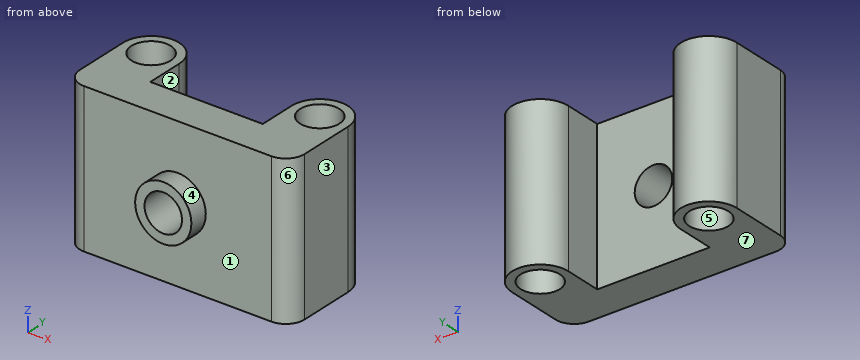
from build123d import *

# Parameters (mm, degrees)
SKETCH_1_W          = 12
SKETCH_1_H          = 8
EXTRUDE_1_DEPTH     = 2
EXTRUDE_6_DEPTH     = 8
SKETCH_11_R         = 1.05
CUT_EXTRUDE_1_DEPTH = 16.43534904
FILLET_3_R          = 1
SKETCH_12_R         = 1
CUT_EXTRUDE_2_DEPTH = 2
EXTRUDE_START       = 1
SKETCH_13_R         = 1.5
SKETCH_13_R_2       = 1
EXTRUDE_7_DEPTH     = 1


with BuildPart() as part:
    # 草图1 → 凸台-拉伸1 (new body)
    with BuildSketch(Plane(origin=(0, 0, 0), x_dir=(1, 0, 0), z_dir=(0, 1, 0))):
        with Locations((6, 0)):
            Rectangle(SKETCH_1_W, SKETCH_1_H)
    extrude(amount=EXTRUDE_1_DEPTH)

    # 草图10 → 凸台-拉伸6 (add)
    with BuildSketch(Plane(origin=(0, 0, -4), x_dir=(-1, 0, 0), z_dir=(0, 0, -1))):
        with BuildLine():
            Line((-12, 2), (-12, 4))
            ThreePointArc((-12, 4), (-10.5, 5.5), (-9, 4))
            Line((-9, 4), (-9, 2))
            Line((-9, 2), (-12, 2))
        make_face()
        with BuildLine():
            Line((-3, 2), (0, 2))
            Line((0, 2), (0, 4))
            ThreePointArc((0, 4), (-1.5, 5.5), (-3, 4))
            Line((-3, 4), (-3, 2))
        make_face()
    extrude(amount=-EXTRUDE_6_DEPTH)

    # 草图11 → 切除-拉伸1 (cut, through all)
    with BuildSketch(Plane(origin=(0, 0, -4), x_dir=(-1, 0, 0), z_dir=(0, 0, -1))):
        with Locations((-1.5, 4)):
            Circle(SKETCH_11_R)
        with Locations((-10.5, 4)):
            Circle(SKETCH_11_R)
    extrude(amount=-CUT_EXTRUDE_1_DEPTH, mode=Mode.SUBTRACT)

    # 圆角3
    fillet_3_edges = [part.edges().sort_by_distance(p)[0] for p in [
        (12, 0, 0),
        (0, 0, 0),
    ]]
    fillet(fillet_3_edges, radius=FILLET_3_R)

    # 草图12 → 切除-拉伸2 (cut)
    with BuildSketch(Plane.XZ):
        with Locations(Location((6, 0, 0), (0, 0, 270))):
            Circle(SKETCH_12_R)
    extrude(amount=-CUT_EXTRUDE_2_DEPTH, mode=Mode.SUBTRACT)

    # 草图13 → 凸台-拉伸7 (add)
    with BuildSketch(Plane.XZ.offset(EXTRUDE_START)):
        with Locations(Location((6, 0, 0), (0, 0, 90))):
            Circle(SKETCH_13_R)
        with Locations(Location((6, 0, 0), (0, 0, 270))):
            Circle(SKETCH_13_R_2, mode=Mode.SUBTRACT)
    extrude(amount=-EXTRUDE_7_DEPTH)


solid = part.part
For this review, take the finished solid that the model builds, in its own axes (mm). Face numbers are marked on the shaded views. A direction names the side the tool comes from. Round coordinates to 2 decimals unless told otherwise and drop trailing zeros. Loops run counter-clockwise (first coordinate to the right, second up) from the corner with the lowest first, then second, coordinate; pieces in that order, holes last. Notation, with made-up numbers: (-21, 78) - (-1, 78) arc R25 cw to (-1, 101) - close; hole circle Ø10 at (23, -25). An arc over 180 degrees is marked (long way). Put each result on its own line as item: value. Start each with the question number.
1. For the marked faces 1, 2 and 3, list the 3-axis set-ups (+Z, -Z, +X, -X, +Y, -Y) from which the entire face can be reached by the end or side of a thin tool; tool diameter is ignored.
2. Consider section D-D on z = -2.75. State the section outline as (x, y) points, plus the area to 3 significant figures.
3. Consider section C-C on y = 2.5. State the section outline as (x, z) points, plus the area to 3 significant figures.
4. Consider section B-B on x = 1.5. State the section outline as (y, z) points.
5. Insertion check: P1, Ø1, axis at x = 5, z = -3, coming from the +Y side; P2, Ø2.5, axis at x = 1.5, y = 4, coming from the -Z side; P3, Ø3, axis at x = 3, z = 1, coming from the -Y side. Each pin has a flat end and moves straight along its axis. Give the tip position at first contact, or say it passes through.
6. Consider section A-A on z = 0. State the section outline as (x, y) points.
7. For probe 1 along Y at (x, z) = (10.5, 0.75); probe 2 along X at (y, z) = (2.25, 2.75); probe 3 along X at (y, z) = (4.5, 3.75), list the stretches that pass through material, from the lowest coordinate up. Write a range as [from, to].
8. Mouldability with a two-part tool opening along X and no side actions: class the marked faces 4, 5, 6 and 7 as +X half, -X half, draft (parallel to the pull), parting line (faces both ways), or undercut.
Result sheet:
1. face 1: -Y
1. face 2: +Z, -Z, +Y
1. face 3: +Z, -Z, +X, +Y, -Y
2. outline: (0, 1) arc R1 ccw to (1, 0) - (11, 0) arc R1 ccw to (12, 1) - (12, 4) arc R1.5 ccw to (9, 4) - (9, 2) - (3, 2) - (3, 4) arc R1.5 ccw to (0, 4) - close; hole circle Ø2.1 at (1.5, 4); hole circle Ø2.1 at (10.5, 4)
2. area: 35.7 mm^2
3. outline: (0, -4) - (3, -4) - (3, 4) - (0, 4) - close; (9, -4) - (12, -4) - (12, 4) - (9, 4) - close
3. area: 48.0 mm^2
4. outline: (0, -4) - (2.95, -4) - (2.95, 4) - (0, 4) - close; (5.05, -4) - (5.5, -4) - (5.5, 4) - (5.05, 4) - close
5. P1: y = 2
5. P2: z = -4
5. P3: y = 0
6. outline: (0, 1) arc R1 ccw to (1, 0) - (4.5, 0) - (4.5, -1) - (5, -1) - (5, 2) - (3, 2) - (3, 4) arc R1.5 ccw to (0, 4) - close; (7, -1) - (7.5, -1) - (7.5, 0) - (11, 0) arc R1 ccw to (12, 1) - (12, 4) arc R1.5 ccw to (9, 4) - (9, 2) - (7, 2) - close; hole circle Ø2.1 at (1.5, 4); hole circle Ø2.1 at (10.5, 4)
7. probe 1: [0, 2.95], [5.05, 5.5]
7. probe 2: [0, 3], [9, 12]
7. probe 3: [0.09, 0.58], [2.42, 2.91], [9.09, 9.58], [11.42, 11.91]
8. face 4: parting line
8. face 5: undercut
8. face 6: +X half
8. face 7: draft
